```python
from build123d import *

# Parameters (mm, degrees)
EXTRUDE1_DEPTH     = 6.5
SKETCH3_R          = 1.1
CUT_EXTRUDE1_DEPTH = 13.395967086
SKETCH5_R          = 4.1
CUT_EXTRUDE2_DEPTH = 24


with BuildPart() as part:
    # Sketch1 → Extrude1 (new body)
    with BuildSketch(Plane.XY):
        with BuildLine():
            Line((-4.6, -8.312039461), (-4.6, 8.312039461))
            ThreePointArc((-4.6, 8.312039461), (0, 9.5), (4.6, 8.312039461))
            Line((4.6, 8.312039461), (4.6, -8.312039461))
            ThreePointArc((4.6, -8.312039461), (0, -9.5), (-4.6, -8.312039461))
        make_face()
    extrude(amount=EXTRUDE1_DEPTH)

    # Sketch3 → Cut-Extrude1 (cut, through all)
    with BuildSketch(Plane.XY.offset(6.5)):
        with Locations((0, 6.715)):
            Circle(SKETCH3_R)
        with Locations((0, -6.715)):
            Circle(SKETCH3_R)
    extrude(amount=-CUT_EXTRUDE1_DEPTH, mode=Mode.SUBTRACT)

    # Sketch5 → Cut-Extrude2 (cut)
    with BuildSketch(Plane(origin=(0, 0, 0), x_dir=(-1, 0, 0), z_dir=(0, 0, -1))):
        Circle(SKETCH5_R)
    extrude(amount=-CUT_EXTRUDE2_DEPTH, mode=Mode.SUBTRACT)


solid = part.part
```
The model under review builds one solid part; all positions refer to its coordinate system, in mm. Coordinates: 2 decimals unless noted, no trailing zeros. Write each loop counter-clockwise with the first axis right and the second up, starting at its lowest first coordinate (ties: lowest second). Pieces come first, ordered by that corner, then holes.
1) We need section B-B on x = 0. State the section outline as (y, z) points (3 decimals), then the cut area to 3 significant figures.
2) We need section C-C on x = 1.5. State the section outline as (y, z) points.
3) To check wall thickness, follow probe 1 along Y at (x, z) = (0.5, 4); probe 2 along X at (y, z) = (-6.75, 4); probe 3 along Y at (x, z) = (0.75, 1.5). State the ranges of each line that lie inside material, in increasing order.
4) The part is to be moulded in two halves that separate along X. For faces 1 (the face through (-4.6, 0, 3)), 2 (the face through (0.1, -9.5, 3.2)), 3 (the face through (0.534, 4.065, 3.204)), say which applies: pulls with the +X half, pulls with the -X half, needs draft (parallel to the pull), parting line crosses it, or undercut.
5) We need section A-A on y = 0. State the section outline as (x, z) points, then the cut area to 3 significant figures.
6) We need section D-D on z = 4. State the section outline as (x, y) points (3 decimals).
7) Clearance check with flat-ended pins moving along their axes: pin 1 Ø3 at (x, y) = (-2, -5) entering from -Z; pin 2 Ø2 at (x, z) = (2.5, 2) entering from -Y. State where each tip first meets the part, or that it passes through.
Answer list:
1. outline: (-9.5, 0) - (-7.815, 0) - (-7.815, 6.5) - (-9.5, 6.5) - close; (-5.615, 0) - (-4.1, 0) - (-4.1, 6.5) - (-5.615, 6.5) - close; (4.1, 0) - (5.615, 0) - (5.615, 6.5) - (4.1, 6.5) - close; (7.815, 0) - (9.5, 0) - (9.5, 6.5) - (7.815, 6.5) - close
1. area: 41.6 mm2
2. outline: (-9.38, 0) - (-3.82, 0) - (-3.82, 6.5) - (-9.38, 6.5) - close; (3.82, 0) - (9.38, 0) - (9.38, 6.5) - (3.82, 6.5) - close
3. probe 1: y = -9.49 to -7.69, -5.74 to -4.07, 4.07 to 5.74, 7.69 to 9.49
3. probe 2: x = -4.6 to -1.1, 1.1 to 4.6
3. probe 3: y = -9.47 to -7.52, -5.91 to -4.03, 4.03 to 5.91, 7.52 to 9.47
4. face 1: pulls with the -X half
4. face 2: parting line crosses it
4. face 3: undercut
5. outline: (-4.6, 0) - (-4.1, 0) - (-4.1, 6.5) - (-4.6, 6.5) - close; (4.1, 0) - (4.6, 0) - (4.6, 6.5) - (4.1, 6.5) - close
5. area: 6.50 mm2
6. outline: (-4.6, -8.312) arc R9.5 ccw to (4.6, -8.312) - (4.6, 8.312) arc R9.5 ccw to (-4.6, 8.312) - close; hole circle Ø8.2 at (0, 0); hole circle Ø2.2 at (0, -6.715); hole circle Ø2.2 at (0, 6.715)
7. pin 1: stops at z = 0
7. pin 2: stops at y = -9.38
